```python
from build123d import *

# Parameters (mm, degrees)
F0_R     = 57.5
F1_DEPTH = 6.6
F2_SIZE  = 3
F3_W     = 17.8
F3_H     = 2
F4_DEPTH = 23.7
F6_DEPTH = 2


with BuildPart() as f1:
    # F0 (on Top) → F1 (new body)
    with BuildSketch(Plane.XY):
        Circle(F0_R)
    extrude(amount=F1_DEPTH)

    # F2
    f2_edges = [f1.edges().sort_by_distance(p)[0] for p in [
        (-57.5, 0, 6.6),
    ]]
    chamfer(f2_edges, length=F2_SIZE)

    # F3 (on face) → F4 (join)
    with BuildSketch(Plane.XY.offset(6.6)):
        Rectangle(F3_W, F3_H)
    extrude(amount=F4_DEPTH)

    # F5 (on face) → F6 (cut, through all)
    with BuildSketch(Plane.XZ.offset(1)):
        with BuildLine():
            Line((8.9, 6.6), (8.9, 21.4))
            ThreePointArc((8.9, 21.4), (6.9052664574, 15.7850828009), (1.8152145724, 12.6870787875))
            Line((1.8152145724, 12.6870787875), (7.0434488575, 6.6))
            Line((7.0434488575, 6.6), (8.9, 6.6))
        make_face()
        with BuildLine():
            ThreePointArc((1.8152145724, 12.6870787875), (6.9052664574, 15.7850828009), (8.9, 21.4))
            ThreePointArc((8.9, 21.4), (8.7734765611, 22.8953625083), (8.3975035885, 24.3482085207))
            ThreePointArc((8.3975035885, 24.3482085207), (8.494665146, 23.9727539281), (8.5273622155, 23.5863119259))
            ThreePointArc((8.5273622155, 23.5863119259), (6.6138042116, 21.3190089943), (4.0572208384, 22.8244153427))
            ThreePointArc((4.0572208384, 22.8244153427), (4.238870699, 22.12247851), (4.3, 21.4))
            ThreePointArc((4.3, 21.4), (1.4939175147, 17.3678528723), (-3.2619583531, 18.5982812949))
            Line((-3.2619583531, 18.5982812949), (1.8152145724, 12.6870787875))
        make_face()
        with BuildLine():
            ThreePointArc((4.3, 21.4), (4.238870699, 22.12247851), (4.0572208384, 22.8244153427))
            ThreePointArc((4.0572208384, 22.8244153427), (-2.1501541462, 25.1238202356), (-3.2619583531, 18.5982812949))
            ThreePointArc((-3.2619583531, 18.5982812949), (1.4939175147, 17.3678528723), (4.3, 21.4))
        make_face()
        with BuildLine():
            ThreePointArc((8.3975035885, 24.3482085207), (8.7734765611, 22.8953625083), (8.9, 21.4))
            Line((8.9, 21.4), (8.9, 30.3))
            Line((8.9, 30.3), (0, 30.3))
            ThreePointArc((0, 30.3), (5.146403801, 28.6611657409), (8.3975035885, 24.3482085207))
        make_face()
        with BuildLine():
            ThreePointArc((-8.9, 21.4), (-6.2932503526, 27.6932503526), (0, 30.3))
            Line((0, 30.3), (-8.9, 30.3))
            Line((-8.9, 30.3), (-8.9, 21.4))
        make_face()
        with BuildLine():
            Line((-2.7928547934, 6.6), (-8.0305968219, 17.5633980289))
            ThreePointArc((-8.0305968219, 17.5633980289), (-8.6799283325, 19.4330622423), (-8.9, 21.4))
            Line((-8.9, 21.4), (-8.9, 6.6))
            Line((-8.9, 6.6), (-2.7928547934, 6.6))
        make_face()
    extrude(amount=-F6_DEPTH, mode=Mode.SUBTRACT)


solid = f1.part
```
Part model, mm, in its own coordinate system. A direction names the side the tool comes from. Give positions to 0.01 mm unless a question says otherwise; leave off trailing zeros. Write each loop counter-clockwise with the first axis right and the second up, starting at its lowest first coordinate (ties: lowest second). Pieces come first, ordered by that corner, then holes. Notation, with made-up numbers: M -27,4 L 3,4 A20 cw 3,14 Z; hole C 66.25,83 d5. An arc over 180 degrees is marked long. Use CSV: the item, a comma, the result in double quotes.
Item 1: Drill centre lines: probe 1 along Z at (x, y) = (-41, 4); probe 2 along X at (y, z) = (0, 21); probe 3 along Z at (x, y) = (0, 0.65). Where is each one in solid material? Low to high.
Taken from the geometry:
probe 1,"z = 0 to 6.6"
probe 2,"x = -8.89 to -4.28"
probe 3,"z = 0 to 14.8, 25.7 to 30.3"
Item 2: Slice it at A-A on z = 10. Write the cut outline in (x, y).
Taken from the geometry:
outline,"M -4.42,-1 L 4.12,-1 L 4.12,1 L -4.42,1 Z"
Item 3: Which spindle directions (+Z, -Z, +X, -X, +Y, -Y) get a long thin tool onto all of the face, cutting with end or side? Do faces 4 (the face through (-4, 1, 18)), 5 (the face through (-4, -1, 18)), 6 (the face through (-12.465, -56.133, 1.775)). Say none if no direction does.
Taken from the geometry:
face 4,"+Z, +X, -X, +Y"
face 5,"+Z, +X, -X, -Y"
face 6,"+Z, -Z"
Item 4: Pin check, flat tips, straight feed: P1, Ø12, axis at x = -0.5, z = 6, coming from the -Y side; P2, Ø10, axis at y = -28.5, z = 10.5, coming from the -X side; P3, Ø11, axis at x = 0, z = 21.4, coming from the -Y side. Stop position of each tip, or through.
Taken from the geometry:
P1,"stops at y = -57.5"
P2,"stops at x = -48.41"
P3,"stops at y = -1"
Item 5: Pull direction X, two halves, no side cores. Call faces 1 (the face through (-7.114, 54.181, 6.454)), 2 (the face through (-1, -11, 6.6)), 3 (the face through (-2.058, -0.014, 25.176)): +X half, -X half, draft (parallel to the pull), parting line (faces both ways), or undercut.
Taken from the geometry:
face 1,"parting line"
face 2,"draft"
face 3,"undercut"
